```python
from build123d import *

# Parameters (mm, degrees)
SKETCH1_W                        = 139.7
SKETCH1_H                        = 152.4
BOSS_EXTRUDE1_DEPTH              = 3.175
SKETCH2_W                        = 3.175
SKETCH2_H                        = 19.05
CUT_EXTRUDE1_DEPTH               = 117.217805292
LPATTERN1_COUNT                  = 11
LPATTERN1_PITCH                  = 13.335
F_13_64_0_20313_DIAMETER_HOLE1_D = 5.159502
LPATTERN2_COUNT                  = 2
LPATTERN2_PITCH                  = 53.34


with BuildPart() as part:
    # Sketch1 → Boss-Extrude1 (new body)
    with BuildSketch(Plane(origin=(0, 0, 0), x_dir=(1, 0, 0), z_dir=(0, 1, 0))):
        with Locations((-9.926173285, 8.252707581)):
            Rectangle(SKETCH1_W, SKETCH1_H)
    extrude(amount=BOSS_EXTRUDE1_DEPTH)

    # Sketch2 → Cut-Extrude1 (cut, through all)
    with BuildSketch(Plane(origin=(0, 3.175, 0), x_dir=(1, 0, 0), z_dir=(0, 1, 0))):
        with Locations((-78.188673285, 62.227707581)):
            Rectangle(SKETCH2_W, SKETCH2_H)
        with Locations((-78.188673285, 8.887707581)):
            Rectangle(SKETCH2_W, SKETCH2_H)
        with Locations((-78.188673285, -44.452292419)):
            Rectangle(SKETCH2_W, SKETCH2_H)
    cut_extrude1 = extrude(amount=-CUT_EXTRUDE1_DEPTH, mode=Mode.SUBTRACT)

    # LPattern1: Cut-Extrude1 ×11
    with Locations(*[(i * LPATTERN1_PITCH, 0, 0) for i in range(1, LPATTERN1_COUNT)]):
        add(cut_extrude1, mode=Mode.SUBTRACT)

    # 13/64 (0.20313) Diameter Hole1 (through all)
    with Locations(Plane(origin=(0, 3.175, 0), x_dir=(1, 0, 0), z_dir=(0, 1, 0))):
        with Locations((55.161326715, -17.782292419), (41.826326715, -17.782292419), (28.491326715, -17.782292419), (15.156326715, -17.782292419), (1.821326715, -17.782292419), (-11.513673285, -17.782292419), (-24.848673285, -17.782292419), (-38.183673285, -17.782292419), (-51.518673285, -17.782292419), (-64.853673285, -17.782292419), (-78.188673285, -17.782292419), (-91.523673285, -17.782292419), (-104.858673285, -17.782292419), (-118.193673285, -17.782292419), (-131.528673285, -17.782292419)):
            f_13_64_0_20313_diameter_hole1 = Hole(F_13_64_0_20313_DIAMETER_HOLE1_D / 2)

    # LPattern2: 13/64 (0.20313) Diameter Hole1 ×2
    with Locations(*[(0, 0, -i * LPATTERN2_PITCH) for i in range(1, LPATTERN2_COUNT)]):
        add(f_13_64_0_20313_diameter_hole1, mode=Mode.SUBTRACT)


solid = part.part
```
Input: part model. Units: mm. Frame: model coordinates. A direction names the side the tool comes from. Coordinates: 2 decimals unless noted, no trailing zeros. Use a Markdown table: item, result. Add a question column.
1) Draft query along Z for faces 4 (the flat face through (-79.776, 2, -26)), 5 (the flat face through (-25, 2, 53.977)). Return one class per face: +Z half, -Z half, draft (parallel to the pull), parting line (faces both ways), or undercut.
2) Set-up query: faces 1 (the flat face through (-53.106, 2, -9)), 2 (the flat face through (-78, 2, 53.977)), 3 (the flat face through (5, 3.175, -9)). Return all of +Z, -Z, +X, -X, +Y, -Y with unobstructed straight access to the full face (end or side cutting, diameter ignored); none if empty.
3) Pin query (flat end, axial travel): P1, Ø4, axis at x = 28.49, z = 17.78, coming from the -Y side; P2, Ø1.6, axis at y = 1, z = 46.5, coming from the -X side. Return the tip coordinate at first contact, or that it passes through.
4) Line query: L1, parallel to Z at x = 54.5, y = 2.9; L2, parallel to Z at x = 28, y = 1.8. Output: solid intervals per line, ascending. Write a range as from..to.
5) Section A-A, the plane z = -57. Give the number of separate pieces and of enclosed holes in the cut face, plus the area to 3 significant figures.
Answer below:
| question | item | result |
|---|---|---|
| 1 | face 4 | draft |
| 1 | face 5 | undercut |
| 2 | face 1 | +Y, -Y |
| 2 | face 2 | -X, +Y, -Y |
| 2 | face 3 | +Z, -Z, +X, -X, +Y |
| 3 | P1 | through |
| 3 | P2 | x = -76.6 |
| 4 | L1 | -84.45..-71.75, -52.7..-38.05, -33.06..-18.41, 0.64..15.29, 20.28..34.93, 53.98..67.95 |
| 4 | L2 | -84.45..-71.75, -52.7..-38.09, -33.03..-18.41, 0.64..15.25, 20.31..34.93, 53.98..67.95 |
| 5 | separate pieces | 11 |
| 5 | enclosed holes | 0 |
| 5 | area | 333 mm2 |
